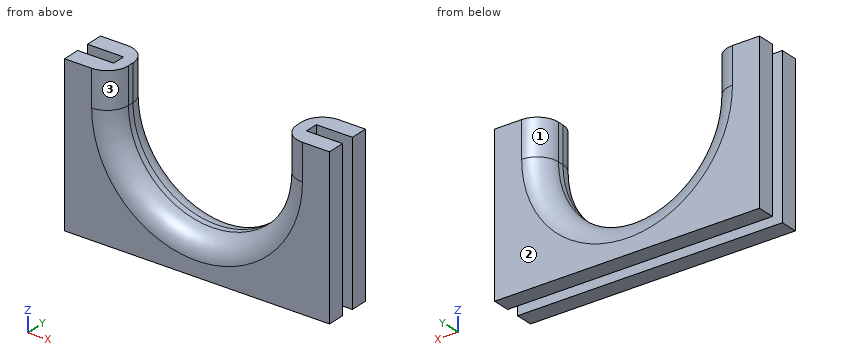
```python
from build123d import *

# Parameters (mm, degrees)
PAD_DEPTH    = 2
POCKET_DEPTH = 0.55
FILLET_R     = 1.75


with BuildPart() as part:
    # Sketch → Pad (new body, symmetric)
    with BuildSketch(Plane.XZ):
        with BuildLine():
            Line((11, 0), (-11, 0))
            Line((-11, 0), (-11, 13))
            Line((-11, 13), (-7, 13))
            Line((-7, 13), (-7, 10))
            ThreePointArc((-7, 10), (0, 3), (7, 10))
            Line((7, 13), (7, 10))
            Line((11, 13), (7, 13))
            Line((11, 13), (11, 0))
        make_face()
    extrude(amount=PAD_DEPTH, both=True)

    # Sketch001 → Pocket (cut, symmetric)
    with BuildSketch(Plane.XZ):
        with BuildLine():
            Line((8, 10), (8, 16))
            Line((8, 16), (12, 16))
            Line((12, 16), (12, 0))
            Line((12, 0), (-12, 0))
            Line((-12, 0), (-12, 16))
            Line((-12, 16), (-8, 16))
            Line((-8, 16), (-8, 10))
            ThreePointArc((-8, 10), (0, 2), (8, 10))
        make_face()
    extrude(amount=POCKET_DEPTH, both=True, mode=Mode.SUBTRACT)

    # Fillet
    fillet_edges = [part.edges().sort_by_distance(p)[0] for p in [
        (0, 2, 3),
        (0, -2, 3),
    ]]
    fillet(fillet_edges, radius=FILLET_R)


solid = part.part
```
Source: CAD feature listing. Evaluate the final solid. Frame: model axes, mm. Face numbers are marked on the shaded views. A direction names the side the tool comes from. Round coordinates to 2 decimals unless told otherwise and drop trailing zeros. Order: outer loops, then holes, each group sorted by start corner. A loop starts at its lowest first (then second) coordinate and runs counter-clockwise, first axis right, second up. Notation, with made-up numbers: (59, 12.5) -> (82, 12.5) arc R10 ccw to (82, 28.5) -> close; hole circle Ø7 at (45, -7). An arc over 180 degrees is marked (long way). Use CSV: the item, a comma, the result in double quotes.
(1) Access query for the marked faces 1, 2 and 3. Directions: +Z, -Z, +X, -X, +Y, -Y. A direction counts if a zero-diameter tool reaches every point of the face in a straight line with its end or side. Return the directions, or none.
Report:
face 1,"+Z, +Y"
face 2,"+Z, -Z, +X, -X, +Y"
face 3,"+Z, -Y"
(2) Section D-D on y = 0.9. Return the cut outline in (x, z), and give its area (3 significant figures).
Report:
outline,"(-11, 0) -> (11, 0) -> (11, 13) -> (7.13, 13) -> (7.13, 10) arc R7.13 cw to (-7.13, 10) -> (-7.13, 13) -> (-11, 13) -> close"
area,"164 mm^2"
(3) Section B-B on y = -1.65. Return the cut outline in (x, z).
Report:
outline,"(-11, 0) -> (11, 0) -> (11, 13) -> (7.7, 13) -> (7.7, 10) arc R7.7 cw to (-7.7, 10) -> (-7.7, 13) -> (-11, 13) -> close"
(4) Section C-C on x = 0. Return the cut outline in (y, z).
Report:
outline,"(-2, 0) -> (-0.55, 0) -> (-0.55, 2) -> (0.55, 2) -> (0.55, 0) -> (2, 0) -> (2, 1.25) arc R1.75 ccw to (0.25, 3) -> (-0.25, 3) arc R1.75 ccw to (-2, 1.25) -> close"
(5) First-contact query: pin 1 Ø0.6 at (y, z) = (0, 11) entering from -X; pin 2 Ø1 at (x, y) = (0.5, 1) entering from +Z; pin 3 Ø5 at (x, z) = (0, 4.5) entering from +Y. Flat tips, straight axial feed; report the tip coordinate or a pass-through.
Report:
pin 1,"x = -8"
pin 2,"z = 3.01"
pin 3,"y = 1.83"
(6) Section A-A on z = 11.5. Return the cut outline in (x, y).
Report:
outline,"(-11, -2) -> (-8.75, -2) arc R1.75 ccw to (-7, -0.25) -> (-7, 0.25) arc R1.75 ccw to (-8.75, 2) -> (-11, 2) -> (-11, 0.55) -> (-8, 0.55) -> (-8, -0.55) -> (-11, -0.55) -> close; (7, -0.25) arc R1.75 ccw to (8.75, -2) -> (11, -2) -> (11, -0.55) -> (8, -0.55) -> (8, 0.55) -> (11, 0.55) -> (11, 2) -> (8.75, 2) arc R1.75 ccw to (7, 0.25) -> close"
(7) Ray query, L1, parallel to Y at x = -5.25, z = 3; L2, parallel to X at y = -0.9, z = 8.75. Return the intervals inside material, ascending.
Report:
L1,"-2 to -0.55, 0.55 to 2"
L2,"-11 to -7.01, 7.01 to 11"
